Work out the finished part from the listing and answer in its coordinate system (mm). Face numbers are marked on the shaded views. Give positions to 0.01 mm unless a question says otherwise; leave off trailing zeros. Loops run counter-clockwise (first coordinate to the right, second up) from the corner with the lowest first, then second, coordinate; pieces in that order, holes last. Notation, with made-up numbers: (86.25, -9.75) - (113.25, -9.75) arc R35 cw to (113.25, 29.25) - close; hole circle Ø6 at (-21, 66.25). An arc over 180 degrees is marked (long way). Use CSV: the item, a comma, the result in double quotes.
from build123d import *

# Parameters (mm, degrees)
F0_W     = 3.175
F0_H     = 127
F0_H_2   = 4.445
F0_H_3   = 3.175
F0_W_2   = 34.925
F1_DEPTH = 12.7
F2_DEPTH = 3.175


# Not quite as in the source:
# - a length typed as a fraction of an inch, garbled in the dataset ("3 / 203.2 mm" for 3/8 in), is restored


with BuildPart() as f1:
    # F0 (on Top) → F1 (new body)
    with BuildSketch(Plane.XY):
        with Locations((-1.5875, 63.5)):
            Rectangle(F0_W, F0_H)
        with Locations((-1.5875, -2.2225)):
            Rectangle(F0_W, F0_H_2)
        with Locations((-1.5875, -6.0325)):
            Rectangle(F0_W, F0_H_3)
        with Locations((17.4625, -6.0325)):
            Rectangle(F0_W_2, F0_H_3)
    extrude(amount=F1_DEPTH)

    # F0 (on Top) → F2 (join)
    with BuildSketch(Plane.XY):
        with Locations((17.4625, -2.2225)):
            Rectangle(F0_W_2, F0_H_2)
    extrude(amount=F2_DEPTH)


solid = f1.part
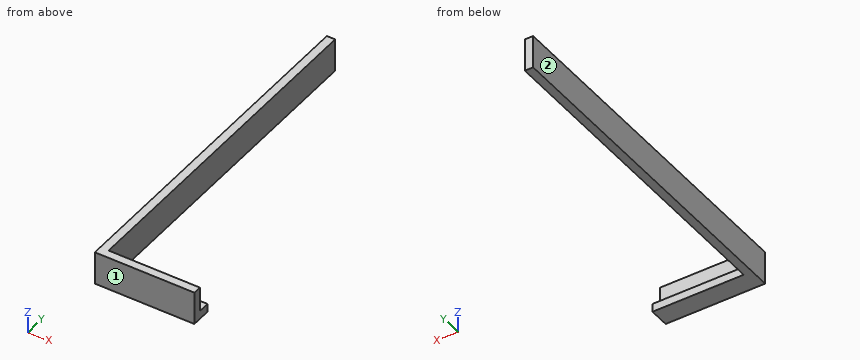
Item 1: A cutting plane is placed at B-B on x = 7. Determine the outline of the cut face in (y, z) (3 decimals).
Determined:
outline,"(-7.62, 0) - (0, 0) - (0, 3.175) - (-4.445, 3.175) - (-4.445, 12.7) - (-7.62, 12.7) - close"
Item 2: A cutting plane is placed at A-A on z = 2. Determine the outline of the cut face in (x, y) (3 decimals), and give its area (3 significant figures).
Determined:
outline,"(-3.175, -7.62) - (34.925, -7.62) - (34.925, 0) - (0, 0) - (0, 127) - (-3.175, 127) - close"
area,"694 mm²"
Item 3: The mould has two halves that part along Y. Classify the marked faces 1 and 2: pulls with the +Y half, pulls with the -Y half, needs draft (parallel to the pull), parting line crosses it, or undercut.
Determined:
face 1,"pulls with the -Y half"
face 2,"needs draft"
Item 4: A cutting plane is placed at C-C on y = 37. Determine the outline of the cut face in (x, z) (3 decimals).
Determined:
outline,"(-3.175, 0) - (0, 0) - (0, 12.7) - (-3.175, 12.7) - close"
Item 5: Find the intervals of material crossed by line 1 (Y direction, x = 23.5, z = 11) (3 decimals); line 2 (X direction, y = 15.5, z = 7.5) (3 decimals); line 3 (Y direction, x = 14, z = 2.5), in increasing order.
Determined:
line 1,"y = -7.62 to -4.445"
line 2,"x = -3.175 to 0"
line 3,"y = -7.62 to 0"
Item 6: Given P1, Ø4, axis at x = 12, z = 6.5, coming from the +Y side (3 decimals); P2, Ø5, axis at y = 71, z = 1.5, coming from the +X side; P3, Ø3.5, axis at x = 26, z = 1, coming from the +Y side, each flat-ended and moving along its own axis, determine where each tip first touches the part or whether it passes through.
Determined:
P1,"stops at y = -4.445"
P2,"stops at x = 0"
P3,"stops at y = 0"
